Model file for the job. Use its own axes, mm. A direction names the side the tool comes from. Give positions to 0.01 mm unless a question says otherwise; leave off trailing zeros. Answer as CSV lines item,"result". Start each with the question number.
Item 1: Drill centre lines: L1, parallel to Y at x = -11, z = 1.85; L2, parallel to X at y = -0.5, z = 2.25; L3, parallel to Y at x = 4, z = 5.3. Where is each one in solid material? Low to high. Write a range as from..to.
Item 2: Saw through at A-A on z = 0.85. State how many separate pieces and enclosed holes the cut face has, plus the area to 3 significant figures.
Item 3: Pin check, flat tips, straight feed: pin 1 (8 mm diameter, centred on x = 26, y = 1, fed in from -Z); pin 2 (4 mm diameter, centred on x = -11, y = 0, fed in from -Z); pin 3 (0.6 mm diameter, centred on y = -8, z = 2, fed in from +X); pin 4 (3 mm diameter, centred on x = -4.5, z = 4, fed in from -Y). Stop position of each tip, or through.
Item 4: Tool access for faces 1 (the flat face through (-2, -5, 3)), 2 (the flat face through (31.937, -6.407, 2.958)), 3 (the cylindrical face through (-16, 0, 3)): list every direction of +Z, -Z, +X, -X, +Y, -Y with a clear straight run to the whole face (end or side of a thin tool).
from build123d import *

# Parameters (mm, degrees)
SKETCH_1_R             = 1.5
EXTRUDE_1_DEPTH        = 6
EXTRUDE_START          = -6
SKETCH_2_R             = 1.5
EXTRUDE_2_DEPTH        = 6
CUT_EXTRUDE_1_DEPTH    = 6
PATTERN_LINEAR_1_COUNT = 9
PATTERN_LINEAR_1_PITCH = 1


with BuildPart() as part:
    # 草图1 → 凸台-拉伸1 (new body)
    with BuildSketch(Plane.XY):
        with BuildLine():
            Line((-11, 5), (11, 5))
            ThreePointArc((11, 5), (16, 0), (11, -5))
            Line((11, -5), (-11, -5))
            ThreePointArc((-11, -5), (-16, 0), (-11, 5))
        make_face()
        with Locations((-11, 0)):
            Circle(SKETCH_1_R, mode=Mode.SUBTRACT)
        with Locations((11, 0)):
            Circle(SKETCH_1_R, mode=Mode.SUBTRACT)
    extrude(amount=EXTRUDE_1_DEPTH)

    # 草图2 → 凸台-拉伸2 (add)
    with BuildSketch(Plane.XY.offset(6).offset(EXTRUDE_START)):
        with BuildLine():
            Line((17.768794041, -2.486649801), (29.011601927, -7.527047167))
            Line((29.011601927, -7.527047167), (34.945301709, -5.255713659))
            Line((34.945301709, -5.255713659), (43.157744395, -8.937531841))
            ThreePointArc((43.157744395, -8.937531841), (37.870669943, -13.928931417), (30.602691257, -13.719857707))
            Line((30.602691257, -13.719857707), (16.032361282, -7.187659205))
            ThreePointArc((16.032361282, -7.187659205), (11.034404004, -5.553031682), (5.805088555, -5))
            Line((5.805088555, -5), (11, -5))
            ThreePointArc((11, -5), (14.590532493, -3.479666135), (15.99754173, 0.156769434))
            ThreePointArc((15.99754173, 0.156769434), (16.503827213, -1.419121599), (17.768794041, -2.486649801))
        make_face()
        with Locations((36.549821691, -11.454545455)):
            Circle(SKETCH_2_R, mode=Mode.SUBTRACT)
    extrude(amount=EXTRUDE_2_DEPTH)

    # 草图3 → 切除-拉伸1 (cut)
    with BuildSketch(Plane.XY.offset(6)):
        Polygon((42.906043034, -8.8246886), (42.496952125, -9.189233202), (42.496952125, -8.641284173), align=None)
    cut_extrude_1 = extrude(amount=-CUT_EXTRUDE_1_DEPTH, mode=Mode.SUBTRACT)

    # 阵列(线性)1: 切除-拉伸1 ×9
    with Locations(*[Vector(-0.9124936318129422, 0.4090909090909094, 0) * (i * PATTERN_LINEAR_1_PITCH) for i in range(1, PATTERN_LINEAR_1_COUNT)]):
        add(cut_extrude_1, mode=Mode.SUBTRACT)


solid = part.part
Responses:
1,L1,"-5..-1.5, 1.5..5"
1,L2,"-15.97..-12.41, -9.59..9.59, 12.41..16.09"
1,L3,"-5..5"
2,separate pieces,"1"
2,enclosed holes,"3"
2,area,"454 mm2"
3,pin 1,"through"
3,pin 2,"z = 0"
3,pin 3,"x = 41.58"
3,pin 4,"y = -5"
4,face 1,"+Z, -Z, -X, -Y"
4,face 2,"+Z, -Z, +Y"
4,face 3,"+Z, -Z, -X"
